Design review of the part shown in the three views and the two pictorial views. Dimensions are in mm from the part's minimum x, y and z. Give positions to 0.01 mm unless a question says otherwise; leave off trailing zeros. Answer as a JSON object with one key per item and string values.
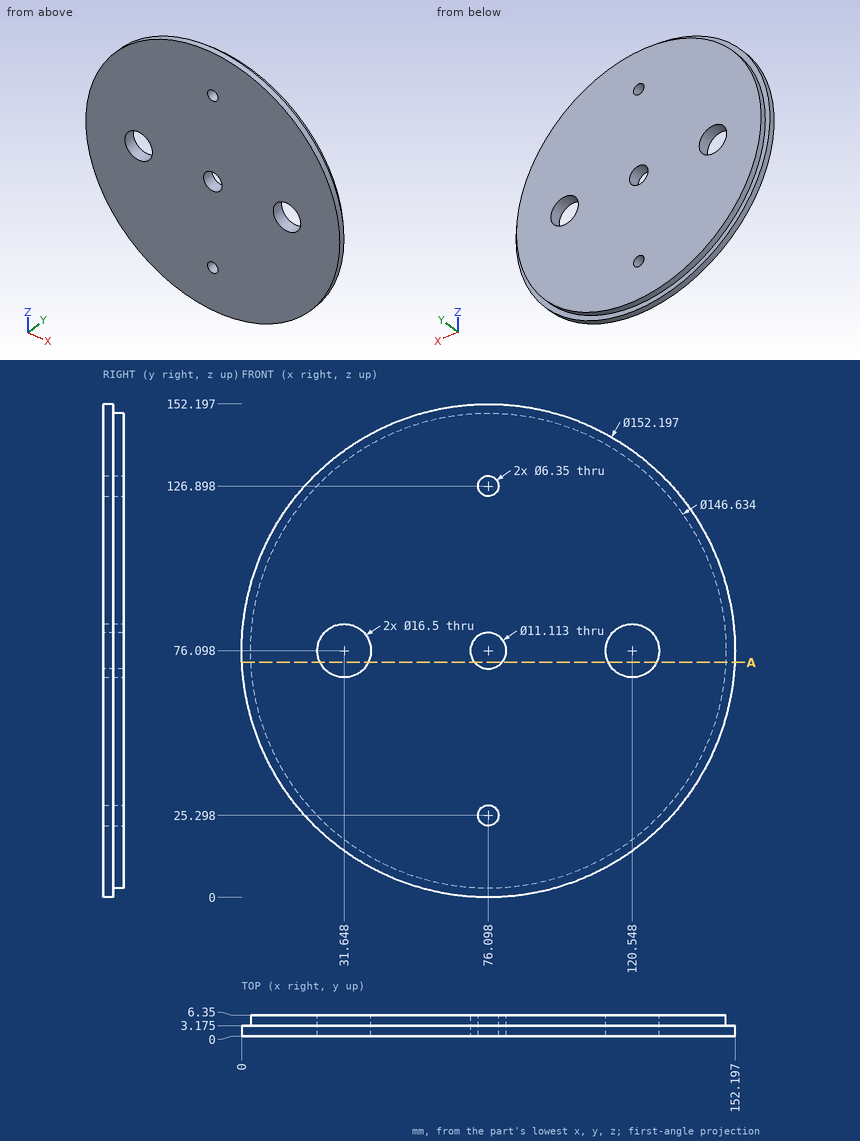
Q1. To check wall thickness, follow probe 1 along X at (y, z) = (2.25, 78.5) (1 decimal); probe 2 along X at (y, z) = (4.5, 75) (1 decimal); probe 3 along Z at (x, y) = (119.5, 5.5) (1 decimal). State the ranges of each line that lie inside material, in increasing order. Write a range as [from, to].
Results:
{"probe 1": "x = [0, 23.8], [39.5, 71.1], [81.1, 112.7], [128.4, 152.2]", "probe 2": "x = [2.8, 23.5], [39.8, 70.7], [81.5, 112.4], [128.7, 149.4]", "probe 3": "z = [17, 67.9], [84.3, 135.2]"}
Q2. Consider section A-A, the plane z = 72.5. State how many separate pieces and enclosed holes the cut face has.
Results:
{"separate pieces": "4", "enclosed holes": "0"}
Q3. Clearance check with flat-ended pins moving along their axes: pin 1 Ø3 at (x, z) = (19, 41) entering from -Y; pin 2 Ø3 at (x, y) = (50.5, 2) entering from -Z; pin 3 Ø2 at (y, z) = (5.5, 110) entering from +X; pin 4 Ø2 at (x, y) = (127.5, 4) entering from +Z (1 decimal). State where each tip first meets the part, or that it passes through.
Results:
{"pin 1": "stops at y = 0", "pin 2": "stops at z = 3.92", "pin 3": "stops at x = 141.62", "pin 4": "stops at z = 132.7"}
